```python
from build123d import *

# Parameters (mm, degrees)
SKETCH2_R               = 3.4925
BOSS_EXTRUDE1_DEPTH     = 101.6
FILLET1_R               = 2.54
CUT_EXTRUDE1_START      = -2.54
SKETCH11_R              = 1
CUT_EXTRUDE1_DEPTH      = 25.246691527
MIRROR3_START           = -2.54
MIRROR3_COPY_1_SKETCH_R = 1
MIRROR3_COPY_1_DEPTH    = 25.246691527
SKETCH12_R              = 3.175
CUT_EXTRUDE2_DEPTH      = 22.706691527
CUT_EXTRUDE2_DEPTH_BACK = 58.627716011
SKETCH13_R              = 3.175
CUT_EXTRUDE3_DEPTH      = 22.706691527
CUT_EXTRUDE3_DEPTH_BACK = 58.627716011
SKETCH14_R              = 3.175
BOSS_EXTRUDE2_DEPTH     = 76.2


with BuildPart() as part:
    # Sketch2 → Boss-Extrude1 (new body)
    with BuildSketch(Plane(origin=(0, 0, 0), x_dir=(1, 0, 0), z_dir=(0, 1, 0))):
        Polygon((19.05, -6.35), (31.75, -6.35), (31.75, 6.35), (19.05, 6.35), (0, 25.4), (-19.05, 6.35), (-31.75, 6.35), (-31.75, -6.35), (-19.05, -6.35), (0, -25.4), align=None)
        Polygon((-19.05, 2.757897552), (0, 21.807897552), (19.05, 2.757897552), (19.05, -2.757897552), (0, -21.807897552), (-19.05, -2.757897552), align=None, mode=Mode.SUBTRACT)
        with Locations((25.4, 0)):
            Circle(SKETCH2_R, mode=Mode.SUBTRACT)
        with Locations((-25.4, 0)):
            Circle(SKETCH2_R, mode=Mode.SUBTRACT)
    extrude(amount=BOSS_EXTRUDE1_DEPTH)

    # Fillet1
    fillet1_edges = [part.edges().sort_by_distance(p)[0] for p in [
        (0, 50.8, 25.4),
        (-19.05, 50.8, 6.35),
        (-31.75, 50.8, 6.35),
        (-31.75, 50.8, -6.35),
        (-19.05, 50.8, -6.35),
        (0, 50.8, -25.4),
        (19.05, 50.8, -6.35),
        (31.75, 50.8, -6.35),
        (31.75, 50.8, 6.35),
        (19.05, 50.8, 6.35),
    ]]
    fillet(fillet1_edges, radius=FILLET1_R)

    # Sketch11 → Cut-Extrude1 (cut)
    with BuildSketch(Plane(origin=(12.7, 0, -12.7), x_dir=(-0.707106781, 0, -0.707106781), z_dir=(0.707106781, 0, -0.707106781)).offset(CUT_EXTRUDE1_START)):
        with Locations((-5.143820715, 5.08)):
            Circle(SKETCH11_R)
        with Locations((12.636179285, 5.08)):
            Circle(SKETCH11_R)
    cut_extrude1 = extrude(amount=CUT_EXTRUDE1_DEPTH, mode=Mode.SUBTRACT)

    # Mirror2: Cut-Extrude1 across plane
    add(cut_extrude1.mirror(Plane(origin=(0, 0, 0), x_dir=(0, 0, 1), z_dir=(1, 0, 0))), mode=Mode.SUBTRACT)

    # Mirror3: Cut-Extrude1 across plane
    add(cut_extrude1.mirror(Plane.XY), mode=Mode.SUBTRACT)

    # Mirror3 copy 1 sketch → Mirror3 copy 1 (cut)
    with BuildSketch(Plane(origin=(-12.7, 0, 12.7), x_dir=(0.707106781, 0, 0.707106781), z_dir=(-0.707106781, 0, 0.707106781)).offset(MIRROR3_START)):
        with Locations((-5.143820715, 5.08)):
            Circle(MIRROR3_COPY_1_SKETCH_R)
        with Locations((12.636179285, 5.08)):
            Circle(MIRROR3_COPY_1_SKETCH_R)
    extrude(amount=MIRROR3_COPY_1_DEPTH, mode=Mode.SUBTRACT)

    # Sketch12 → Cut-Extrude2 (cut, two sides)
    with BuildSketch(Plane(origin=(-12.7, 0, -12.7), x_dir=(-0.707106781, 0, 0.707106781), z_dir=(-0.707106781, 0, -0.707106781))) as cut_extrude2_sk:
        with Locations((0, 76.2)):
            Circle(SKETCH12_R)
    extrude(amount=CUT_EXTRUDE2_DEPTH, mode=Mode.SUBTRACT)
    extrude(cut_extrude2_sk.sketch, amount=-CUT_EXTRUDE2_DEPTH_BACK, mode=Mode.SUBTRACT)

    # Sketch13 → Cut-Extrude3 (cut, two sides)
    with BuildSketch(Plane(origin=(12.7, 0, -12.7), x_dir=(-0.707106781, 0, -0.707106781), z_dir=(0.707106781, 0, -0.707106781))) as cut_extrude3_sk:
        with Locations((0, 63.5)):
            Circle(SKETCH13_R)
    extrude(amount=CUT_EXTRUDE3_DEPTH, mode=Mode.SUBTRACT)
    extrude(cut_extrude3_sk.sketch, amount=-CUT_EXTRUDE3_DEPTH_BACK, mode=Mode.SUBTRACT)

    # Sketch14 → Boss-Extrude2 (add)
    with BuildSketch(Plane(origin=(0, 101.6, 0), x_dir=(1, 0, 0), z_dir=(0, 1, 0))):
        with BuildLine():
            Line((8.980256121, -12.827641431), (0, -21.807897552))
            Line((0, -21.807897552), (-8.980256121, -12.827641431))
            ThreePointArc((-8.980256121, -12.827641431), (0, -9.107897552), (8.980256121, -12.827641431))
        make_face()
        with Locations((0, -14.187897552)):
            Circle(SKETCH14_R, mode=Mode.SUBTRACT)
    extrude(amount=-BOSS_EXTRUDE2_DEPTH)


solid = part.part
```
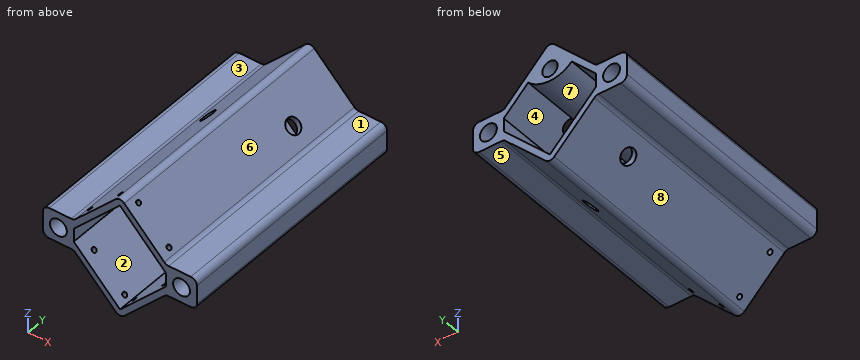
CAD build for the part. Positions are in the model's coordinates, mm. Face numbers are marked on the shaded views. A direction names the side the tool comes from. Coordinates: 2 decimals unless noted, no trailing zeros. Loops run counter-clockwise (first coordinate to the right, second up) from the corner with the lowest first, then second, coordinate; pieces in that order, holes last. Notation, with made-up numbers: (2, 14.25) - (7, 14.25) arc R20 ccw to (7, 24.25) - close; hole circle Ø1 at (20.5, 53). An arc over 180 degrees is marked (long way). Return JSON: item names as keys, results as strings.
1. Probe L1, parallel to Z at x = 0, y = 54.5; L2, parallel to Z at x = 25, y = 51; L3, parallel to X at y = 5, z = 2. List the from-to ranges inside material, lowest first. Write a range as from..to.
Result:
{"L1": "z = -24.35..-21.81, 9.11..11.01, 17.36..24.35", "L2": "z = -6.35..-3.47, 3.47..6.35", "L3": "x = -31.75..-28.26, -22.54..-19.05, 19.05..22.54, 28.26..31.75"}
2. Band-saw the part on B-B (x = 25.4). Give the cut face in (y, z), and give its area (3 significant figures).
Result:
{"outline": "(0, -6.35) - (101.6, -6.35) - (101.6, -3.49) - (0, -3.49) - close; (0, 3.49) - (101.6, 3.49) - (101.6, 6.35) - (0, 6.35) - close", "area": "581 mm2"}
3. Mould opens along X. For the marked faces 6, 7 and 8 say: released by +X, released by -X, zero draft, split by the parting line, or undercut.
Result:
{"face 6": "released by +X", "face 7": "undercut", "face 8": "released by -X"}
4. 3-axis set-ups, long thin cutter, end or side, ignore diameter. For the marked faces 1, 2, 3, 4 and 5: which of +Z, -Z, +X, -X, +Y, -Y reach the whole face in a straight line?
Result:
{"face 1": "+Z, +X, +Y, -Y", "face 2": "+Y, -Y", "face 3": "+Z, -X, +Y, -Y", "face 4": "-Y", "face 5": "-Z, +X, +Y, -Y"}
5. Drop flat-ended pins along their axis: pin 1 (6.5 mm diameter, centred on x = -25.4, z = 0, fed in from -Y); pin 2 (2.5 mm diameter, centred on x = -24.5, y = 40, fed in from -Z); pin 3 (2.5 mm diameter, centred on x = -24, y = 31, fed in from +Z); pin 4 (12 mm diameter, centred on x = -21.5, y = 26, fed in from -Z). Give the stop position or say it passes through.
Result:
{"pin 1": "passes through", "pin 2": "stops at z = -6.35", "pin 3": "stops at z = 6.35", "pin 4": "stops at z = -9.9"}
6. Band-saw the part on C-C (z = 16). Give the cut face in (x, y).
Result:
{"outline": "(-9.4, 0) - (-5.81, 0) - (-5.81, 25.4) - (-2.61, 25.4) - (-2.61, 101.6) - (-9.4, 101.6) - close; (2.61, 25.4) - (5.81, 25.4) - (5.81, 0) - (9.4, 0) - (9.4, 101.6) - (2.61, 101.6) - close"}
7. Band-saw the part on A-A (z = 0). Give the cut face in (x, y), and give its area (3 significant figures).
Result:
{"outline": "(-31.75, 0) - (-28.89, 0) - (-28.89, 101.6) - (-31.75, 101.6) - close; (-21.91, 0) - (-19.05, 0) - (-19.05, 101.6) - (-21.91, 101.6) - close; (19.05, 0) - (21.91, 0) - (21.91, 101.6) - (19.05, 101.6) - close; (28.89, 0) - (31.75, 0) - (31.75, 101.6) - (28.89, 101.6) - close", "area": "1,160 mm2"}
8. Band-saw the part on D-D (y = 51). State how many separate pieces and enclosed holes the cut face has, and give its area (3 significant figures).
Result:
{"separate pieces": "1", "enclosed holes": "4", "area": "607 mm2"}
